Work out the finished part from the listing and answer in its coordinate system (mm). Coordinates: 2 decimals unless noted, no trailing zeros. Loops run counter-clockwise (first coordinate to the right, second up) from the corner with the lowest first, then second, coordinate; pieces in that order, holes last. Notation, with made-up numbers: (35.25, -24.75) - (89.25, -24.75) arc R24 ccw to (89.25, -5.75) - close; hole circle Ø7 at (49.5, 60). An arc over 180 degrees is marked (long way). Write each question's results on one line, items separated by ' | '. Start each with the question number.
Item 1: Each of these flat-tipped pins is pushed along its axis until it touches: pin 1 Ø11.5 at (x, z) = (110.71, 232.5) entering from -Y; pin 2 Ø1.6 at (x, y) = (-4.5, -2) entering from -Z; pin 3 Ø5.5 at (x, z) = (342.71, 50.5) entering from -Y. Where does it stop, or does it pass through?
Item 2: Consider probe 1 along X at (y, z) = (-1.3, 50.5); probe 2 along X at (y, z) = (-0.9, 178); probe 3 along Z at (x, y) = (263.5, -0.6). Determine where each line is inside the solid, lowest interval first. Write a range as [from, to].
Item 3: Section A-A, the plane z = 22.5 is taken. Write down the section's boundary in (x, y), plus the area to 3 significant figures.
Item 4: Section B-B, the plane y = -0.9 is taken. Count the separate pieces of the cut face and the enclosed holes in it, plus the area to 3 significant figures.
Item 5: Section C-C, the plane z = 70.5 is taken. Write down the section's boundary in (x, y), plus the area to 3 significant figures.
Item 6: For a pull along X with two mould halves and no side action, classify faces 1 (the face through (-4.157, -1.563, 229.504)), 2 (the face through (180, 0, 124)) as +X half, -X half, draft (parallel to the pull), parting line (faces both ways), or undercut.
from build123d import *

# Parameters (mm, degrees)
SKETCH1_R           = 4
SKETCH1_R_2         = 3.5
SKETCH1_R_3         = 5
BOSS_EXTRUDE1_DEPTH = 3.17


with BuildPart() as part:
    # Sketch1 → Boss-Extrude1 (new body)
    with BuildSketch(Plane(origin=(0, 0, 0), x_dir=(1, 0, 0), z_dir=(0, 1, 0))):
        Polygon((1.713446604, -2.5), (366.713446604, -2.5), (366.713446604, -248.5), (-12.286553396, -248.5), (-12.286553396, -218.5), (1.713446604, -218.5), align=None)
        with Locations(Location((-4.333354101, -233.5, 0), (0, 0, 270))):
            Circle(SKETCH1_R, mode=Mode.SUBTRACT)
        with Locations(Location((56.754069102, -229.789646053, 0), (0, 0, 270))):
            Circle(SKETCH1_R, mode=Mode.SUBTRACT)
        with Locations(Location((53.713446604, -50.5, 0), (0, 0, 270))):
            Circle(SKETCH1_R_2, mode=Mode.SUBTRACT)
        with Locations(Location((53.713446604, -204.5, 0), (0, 0, 270))):
            Circle(SKETCH1_R_2, mode=Mode.SUBTRACT)
        with Locations(Location((342.713446604, -204.5, 0), (0, 0, 270))):
            Circle(SKETCH1_R_2, mode=Mode.SUBTRACT)
        with Locations(Location((342.713446604, -50.5, 0), (0, 0, 270))):
            Circle(SKETCH1_R_2, mode=Mode.SUBTRACT)
        with Locations(Location((263.133334245, -22.5, 0), (0, 0, 270))):
            Circle(SKETCH1_R_3, mode=Mode.SUBTRACT)
        with Locations(Location((172.713446604, -232.5, 0), (0, 0, 270))):
            Circle(SKETCH1_R_3, mode=Mode.SUBTRACT)
        with Locations(Location((110.713446604, -232.5, 0), (0, 0, 270))):
            Circle(SKETCH1_R_3, mode=Mode.SUBTRACT)
        with Locations(Location((174.553221886, -22.5, 0), (0, 0, 270))):
            Circle(SKETCH1_R_3, mode=Mode.SUBTRACT)
        with Locations(Location((351.713446604, -22.5, 0), (0, 0, 270))):
            Circle(SKETCH1_R_3, mode=Mode.SUBTRACT)
    extrude(amount=-BOSS_EXTRUDE1_DEPTH)


solid = part.part
Answer key:
1) pin 1: stops at y = -3.17 | pin 2: stops at z = 218.5 | pin 3: passes through
2) probe 1: x = [1.71, 50.21], [57.21, 339.21], [346.21, 366.71] | probe 2: x = [1.71, 366.71] | probe 3: z = [2.5, 17.51], [27.49, 248.5]
3) outline: (1.71, -3.17) - (169.55, -3.17) - (169.55, 0) - (1.71, 0) - close; (179.55, -3.17) - (258.13, -3.17) - (258.13, 0) - (179.55, 0) - close; (268.13, -3.17) - (346.71, -3.17) - (346.71, 0) - (268.13, 0) - close; (356.71, -3.17) - (366.71, -3.17) - (366.71, 0) - (356.71, 0) - close | area: 1,060 mm^2
4) separate pieces: 1 | enclosed holes: 11 | area: 89,600 mm^2
5) outline: (1.71, -3.17) - (366.71, -3.17) - (366.71, 0) - (1.71, 0) - close | area: 1,160 mm^2
6) face 1: undercut | face 2: draft
